Part model, mm, in its own coordinate system. A direction names the side the tool comes from. Coordinates: 2 decimals unless noted, no trailing zeros. Loops run counter-clockwise (first coordinate to the right, second up) from the corner with the lowest first, then second, coordinate; pieces in that order, holes last. Notation, with made-up numbers: M 61.25,-30 L 108.25,-30 A21 ccw 108.25,-19 Z; hole C 12,66.25 d5. An arc over 180 degrees is marked long. Use a Markdown table: item, result. Add a question column.
1) Band-saw the part on A-A (x = 0). List the corners of the cut face in (y, z), plus the area to 3 significant figures.
2) Wall check: probe 1 along Y at (x, z) = (0, 6); probe 2 along Y at (x, z) = (0, 13). Give the ranges that are in metal, low to high. Write a range as from..to.
3) Pull direction X, two halves, no side cores. Call faces 3 (the conical face through (2.74, 12.36, 12.16)), 4 (the flat face through (-3, 3, 0)), 5 (the conical face through (-5.678, -1.788, 18.953)), 6 (the cylindrical face through (3, 0, 10)): released by +X, released by -X, zero draft, split by the parting line, or undercut.
4) Band-saw the part on C-C (z = 3). List the corners of the cut face in (x, y).
5) Pin check, flat tips, straight feed: pin 1 Ø4 at (y, z) = (8.5, 10) entering from +X; pin 2 Ø2 at (y, z) = (-8.5, 13.5) entering from +X; pin 3 Ø3 at (x, z) = (0.5, 13.5) entering from +Y; pin 4 Ø12 at (x, y) = (4, -2) entering from +Z. Stop position of each tip, or through.
6) Tool access for faces 1 (the cylindrical face through (-11.923, -3.755, 5.916)), 2 (the flat face through (2.5, 2.5, 18.75)): list every direction of +Z, -Z, +X, -X, +Y, -Y with a clear straight run to the whole face (end or side of a thin tool).
from build123d import *


with BuildPart() as part:
    # Sketch → Revolution (revolve)
    with BuildSketch(Plane.XZ):
        Polygon((-3, 18.75), (-5.75, 18.75), (-9, 22), (-15.75, 15.25), (-12.5, 12), (-12.5, 0), (-3, 0), align=None)
    revolve(axis=Axis((0, 0, 0), (0, 0, 1)))


solid = part.part
Entries:
| question | item | result |
|---|---|---|
| 1 | outline | M -15.75,15.25 L -12.5,12 L -12.5,0 L -3,0 L -3,18.75 L -5.75,18.75 L -9,22 Z; M 3,0 L 12.5,0 L 12.5,12 L 15.75,15.25 L 9,22 L 5.75,18.75 L 3,18.75 Z |
| 1 | area | 398 mm2 |
| 2 | probe 1 | -12.5..-3, 3..12.5 |
| 2 | probe 2 | -13.5..-3, 3..13.5 |
| 3 | face 3 | split by the parting line |
| 3 | face 4 | zero draft |
| 3 | face 5 | undercut |
| 3 | face 6 | undercut |
| 4 | outline | C 0,0 d25; hole C 0,0 d6 |
| 5 | pin 1 | x = 10.68 |
| 5 | pin 2 | x = 12.53 |
| 5 | pin 3 | y = 15.49 |
| 5 | pin 4 | z = 22 |
| 6 | face 1 | -Z |
| 6 | face 2 | +Z |
